from build123d import *

# Parameters (mm, degrees)
SKETCH1_W             = 35
SKETCH1_H             = 35
BOSS_EXTRUDE1_DEPTH   = 20
SKETCH2_W             = 35
SKETCH2_H             = 7
BOSS_EXTRUDE2_DEPTH   = 27
SKETCH3_R             = 8.5
CUT_EXTRUDE1_DEPTH    = 20
CUT_EXTRUDE3_REACH    = 22
SKETCH7_W             = 35
SKETCH7_H             = 5
SKETCH9_W             = 7
SKETCH9_H             = 27
CUT_EXTRUDE4_DEPTH    = 40
M3_TAPPED_HOLE3_D     = 2.5
M3_TAPPED_HOLE3_DEPTH = 7.5
M3_TAPPED_HOLE3_TIP   = 0.751075774


with BuildPart() as part:
    # Sketch1 → Boss-Extrude1 (new body)
    with BuildSketch(Plane(origin=(0, 0, 0), x_dir=(1, 0, 0), z_dir=(0, 1, 0))):
        Rectangle(SKETCH1_W, SKETCH1_H)
    extrude(amount=BOSS_EXTRUDE1_DEPTH)

    # Sketch2 → Boss-Extrude2 (add)
    with BuildSketch(Plane(origin=(0, 20, 0), x_dir=(1, 0, 0), z_dir=(0, 1, 0))):
        with Locations((0, 14)):
            Rectangle(SKETCH2_W, SKETCH2_H)
    extrude(amount=BOSS_EXTRUDE2_DEPTH)

    # Sketch3 → Cut-Extrude1 (cut)
    with BuildSketch(Plane.XZ):
        Circle(SKETCH3_R)
    extrude(amount=-CUT_EXTRUDE1_DEPTH, mode=Mode.SUBTRACT)

    # Sketch7 → Cut-Extrude3 (cut, up to next)
    with BuildSketch(Plane(origin=(0, 20, 0), x_dir=(1, 0, 0), z_dir=(0, 1, 0)), mode=Mode.PRIVATE) as cut_extrude3_sk1:
        with Locations((0, -15)):
            Rectangle(SKETCH7_W, SKETCH7_H)
    cut_extrude3_tool1 = extrude(cut_extrude3_sk1.sketch, amount=-CUT_EXTRUDE3_REACH, mode=Mode.PRIVATE) & part.part
    add(cut_extrude3_tool1.solids().sort_by_distance((0, 20, 15))[0], mode=Mode.SUBTRACT)

    # Sketch9 → Cut-Extrude4 (cut)
    with BuildSketch(Plane.ZY.offset(17.5)):
        with Locations((-14, 33.5)):
            Rectangle(SKETCH9_W, SKETCH9_H)
    extrude(amount=-CUT_EXTRUDE4_DEPTH, mode=Mode.SUBTRACT)

    # M3 Tapped Hole3
    with Locations(Plane(origin=(0, 0, 0), x_dir=(-1, 0, 0), z_dir=(0, -1, 0))):
        with Locations((12.5, 5.5), (-12.5, 5.5), (-12.5, -9.5), (12.5, -9.5)):
            Hole(M3_TAPPED_HOLE3_D / 2, depth=M3_TAPPED_HOLE3_DEPTH)
            with Locations((0, 0, -(M3_TAPPED_HOLE3_DEPTH + M3_TAPPED_HOLE3_TIP / 2))):  # 118° drill point
                Cone(0, M3_TAPPED_HOLE3_D / 2, M3_TAPPED_HOLE3_TIP, mode=Mode.SUBTRACT)


solid = part.part
Source: CAD feature listing. Evaluate the final solid. Frame: model axes, mm. A direction names the side the tool comes from. Give positions to 0.01 mm unless a question says otherwise; leave off trailing zeros. Order: outer loops, then holes, each group sorted by start corner. A loop starts at its lowest first (then second) coordinate and runs counter-clockwise, first axis right, second up. Notation, with made-up numbers: (46, 63) -> (71, 63) arc R27 cw to (71, 97) -> close; hole circle Ø4 at (-1.5, -36). An arc over 180 degrees is marked (long way). Write item = value, one per line.
Q1. Material intervals for line 1 (Z direction, x = -12.5, y = 4); line 2 (X direction, y = 2.5, z = 9.5); line 3 (Z direction, x = -12, y = 6), sorted ascending. Write a range as from..to.
Data:
line_1 = -17.5..-6.75, -4.25..8.25, 10.75..12.5
line_2 = -17.5..-13.75, -11.25..11.25, 13.75..17.5
line_3 = -17.5..-6.65, -4.35..8.35, 10.65..12.5
Q2. Set-up query: faces 1 (the face through (-17.5, 10, -2)), 2 (the face through (11.579, 3.802, 8.655)). Return all of +Z, -Z, +X, -X, +Y, -Y with unobstructed straight access to the full face (end or side cutting, diameter ignored); none if empty.
Data:
face_1 = +Z, -Z, -X, +Y, -Y
face_2 = -Y
Q3. Cut plane C-C, the plane x = 0. Output: boundary loops of the cut face in (y, z).
Data:
outline = (0, -17.5) -> (20, -17.5) -> (20, -8.5) -> (0, -8.5) -> close; (0, 8.5) -> (20, 8.5) -> (20, 12.5) -> (0, 12.5) -> close
Q4. Cut plane D-D, the plane y = 11. Output: boundary loops of the cut face in (x, z).
Data:
outline = (-17.5, -17.5) -> (17.5, -17.5) -> (17.5, 12.5) -> (-17.5, 12.5) -> close; hole circle Ø17 at (0, 0)
Q5. Pull-direction query (Z, two-part tool) for faces 3 (the face through (0, 10, 12.5)), 4 (the face through (17.5, 10, -2)), 5 (the face through (-12.472, 8.121, 9.285)); classes: released by +Z, released by -Z, zero draft, split by the parting line, or undercut.
Data:
face_3 = released by +Z
face_4 = zero draft
face_5 = undercut
Q6. Cut plane B-B, the plane y = 4. Output: boundary loops of the cut face in (x, z), and give its area (3 significant figures).
Data:
outline = (-17.5, -17.5) -> (17.5, -17.5) -> (17.5, 12.5) -> (-17.5, 12.5) -> close; hole circle Ø2.5 at (-12.5, -5.5); hole circle Ø2.5 at (-12.5, 9.5); hole circle Ø17 at (0, 0); hole circle Ø2.5 at (12.5, -5.5); hole circle Ø2.5 at (12.5, 9.5)
area = 803 mm^2
Q7. Cut plane A-A, the plane z = 0. Output: boundary loops of the cut face in (x, y), and give its area (3 significant figures).
Data:
outline = (-17.5, 0) -> (-8.5, 0) -> (-8.5, 20) -> (-17.5, 20) -> close; (8.5, 0) -> (17.5, 0) -> (17.5, 20) -> (8.5, 20) -> close
area = 360 mm^2
Q8. Pin query (flat end, axial travel): pin 1 (1.5 mm diameter, centred on x = -3.5, z = 6, fed in from +Y); pin 2 (2 mm diameter, centred on x = 12.5, z = 9.5, fed in from -Y); pin 3 (3 mm diameter, centred on x = -12.5, z = -5.5, fed in from -Y). Return the tip coordinate at first contact, or that it passes through.
Data:
pin_1 = through
pin_2 = 7.65
pin_3 = 0
